Geometry: final body of the model. Coordinates: model frame, mm. Face numbers are marked on the shaded views. Round coordinates to 2 decimals unless told otherwise and drop trailing zeros. Order: outer loops, then holes, each group sorted by start corner. A loop starts at its lowest first (then second) coordinate and runs counter-clockwise, first axis right, second up. Notation, with made-up numbers: M -31,73 L 5,73 A14 ccw 5,99 Z; hole C -38,55 d11. An arc over 180 degrees is marked long. Return JSON: item names as keys, results as strings. Group by question number.
Q1. Cut plane A-A on x = 25.4. Output: boundary loops of the cut face in (y, z).
Q2. Cut plane C-C on y = 6.75. Count the separate pieces of the cut face and the enclosed holes in it, and give its area (3 significant figures).
Q3. Ray query, probe 1 along X at (y, z) = (13, 1.75) (3 decimals); probe 2 along Z at (x, y) = (38.1, 3.75); probe 3 along Y at (x, z) = (9.5, 1). Return the intervals inside material, ascending.
Q4. Contact query for flat-ended pins moving along their axis: pin 1 (8.5 mm diameter, centred on x = 12.7, y = 6.35, fed in from -Z); pin 2 (2 mm diameter, centred on y = 3.5, z = 0.5, fed in from -X); pin 3 (1.5 mm diameter, centred on x = 11, z = 2, fed in from +Y) (3 decimals). Output: stop coordinate, or through.
Q5. Mould query, pull axis X, two halves, no side actions, for the marked faces 1, 2, 3 and 4. Classes: released by +X, released by -X, zero draft, split by the parting line, or undercut.
Q6. Cut plane B-B on z = 4. Output: boundary loops of the cut face in (x, y) (3 decimals), and give its area (3 significant figures).
```python
from build123d import *

# Parameters (mm, degrees)
F0_R     = 5.207
F1_DEPTH = 6.35
F3_D     = 3.175


with BuildPart() as f1:
    # F0 (on Top) → F1 (new body)
    with BuildSketch(Plane.XY):
        with BuildLine():
            ThreePointArc((15.24, 15.24), (26.0163073453, 10.7763073453), (30.48, 0))
            Line((30.48, 0), (41.275, 0))
            Line((41.275, 0), (41.275, 15.24))
            Line((41.275, 15.24), (15.24, 15.24))
        make_face()
        with BuildLine():
            ThreePointArc((15.24, 15.24), (4.4636926547, 10.7763073453), (0, 0))
            Line((0, 0), (30.48, 0))
            ThreePointArc((30.48, 0), (26.0163073453, 10.7763073453), (15.24, 15.24))
        make_face()
        with Locations((12.7, 6.3490347266)):
            Circle(F0_R, mode=Mode.SUBTRACT)
    extrude(amount=F1_DEPTH)

    # F3 (through all)
    with Locations(Plane.XZ):
        with Locations((25.4, 3.175), (38.1, 3.175)):
            Hole(F3_D / 2)


solid = f1.part
```
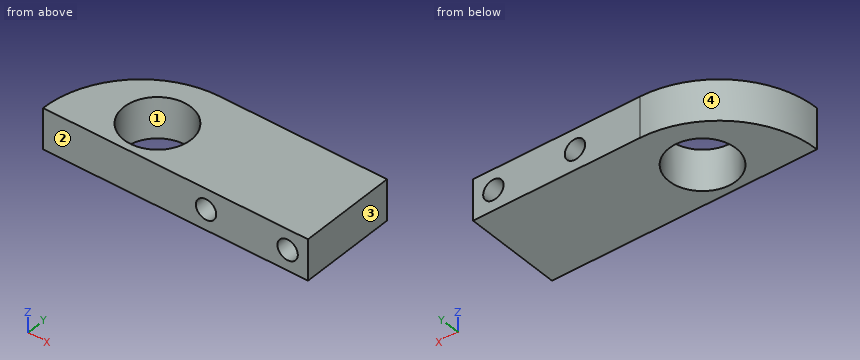
Result sheet:
{
 "1": {"outline": "M 0,0 L 15.24,0 L 15.24,1.59 L 0,1.59 Z; M 0,4.76 L 15.24,4.76 L 15.24,6.35 L 0,6.35 Z"},
 "2": {"separate pieces": "2", "enclosed holes": "2", "area": "170 mm²"},
 "3": {"probe 1": "x = 7.287 to 24.7, 26.1 to 37.4, 38.8 to 41.275", "probe 2": "z = 0 to 1.59, 4.76 to 6.35", "probe 3": "y = 0 to 2.24, 10.46 to 14.12"},
 "4": {"pin 1": "passes through", "pin 2": "stops at x = 0.21", "pin 3": "stops at y = 14.835"},
 "5": {"face 1": "undercut", "face 2": "zero draft", "face 3": "released by +X", "face 4": "released by -X"},
 "6": {"outline": "M 0,0 L 24.044,0 L 24.044,15.24 L 15.24,15.24 A15.24 ccw Z; M 26.756,0 L 36.744,0 L 36.744,15.24 L 26.756,15.24 Z; M 39.456,0 L 41.275,0 L 41.275,15.24 L 39.456,15.24 Z; hole C 12.7,6.349 d10.414", "area": "411 mm²"}
}
